from build123d import *

# Parameters (mm, degrees)
EXTRUDE_1_DEPTH     = 3
SKETCH_3_W          = 25
SKETCH_3_H          = 25
CUT_EXTRUDE_1_DEPTH = 391.157969373
SKETCH_5_R          = 1.5
CUT_EXTRUDE_3_DEPTH = 391.157969373
FILLET_2_R          = 10
SKETCH_6_R          = 1.5
CUT_EXTRUDE_6_DEPTH = 10
SKETCH_7_R          = 1.5
CUT_EXTRUDE_7_DEPTH = 391.157969373


with BuildPart() as part:
    # 草图1 → 凸台-拉伸1 (new body)
    with BuildSketch(Plane.XY):
        Polygon((0, -137.801455237), (0, 0), (-365, 0), (-365, -40), align=None)
    extrude(amount=EXTRUDE_1_DEPTH)

    # 草图3 → 切除-拉伸1 (cut, through all)
    with BuildSketch(Plane.XY.offset(3)):
        with Locations((-12.5, -12.5)):
            Rectangle(SKETCH_3_W, SKETCH_3_H)
    extrude(amount=-CUT_EXTRUDE_1_DEPTH, mode=Mode.SUBTRACT)

    # 草图5 → 切除-拉伸3 (cut, through all)
    with BuildSketch(Plane.XY.offset(3)):
        with Locations((-305, -7)):
            Circle(SKETCH_5_R)
        with Locations((-185, -7)):
            Circle(SKETCH_5_R)
        with Locations((-65, -7)):
            Circle(SKETCH_5_R)
    extrude(amount=-CUT_EXTRUDE_3_DEPTH, mode=Mode.SUBTRACT)

    # 圆角2
    fillet_2_edges = [part.edges().sort_by_distance(p)[0] for p in [
        (0, -25, 1.5),
        (-25, -25, 1.5),
        (-25, 0, 1.5),
    ]]
    fillet(fillet_2_edges, radius=FILLET_2_R)

    # 草图6 → 切除-拉伸6 (cut)
    with BuildSketch(Plane.XY.offset(3)):
        with Locations((-38.637033052, -119.16648399)):
            Circle(SKETCH_6_R)
        with Locations((-67.61480784, -111.401912637)):
            Circle(SKETCH_6_R)
        with Locations((-251.140714835, -62.226294067)):
            Circle(SKETCH_6_R)
        with Locations((-280.118489624, -54.461722714)):
            Circle(SKETCH_6_R)
    extrude(amount=-CUT_EXTRUDE_6_DEPTH, mode=Mode.SUBTRACT)

    # 草图7 → 切除-拉伸7 (cut, through all)
    with BuildSketch(Plane.XY.offset(3)):
        with Locations((-26.327035604, -95.030119084)):
            Circle(SKETCH_7_R)
        with Locations((-16.086178306, -77.850921146)):
            Circle(SKETCH_7_R)
    extrude(amount=-CUT_EXTRUDE_7_DEPTH, mode=Mode.SUBTRACT)


solid = part.part
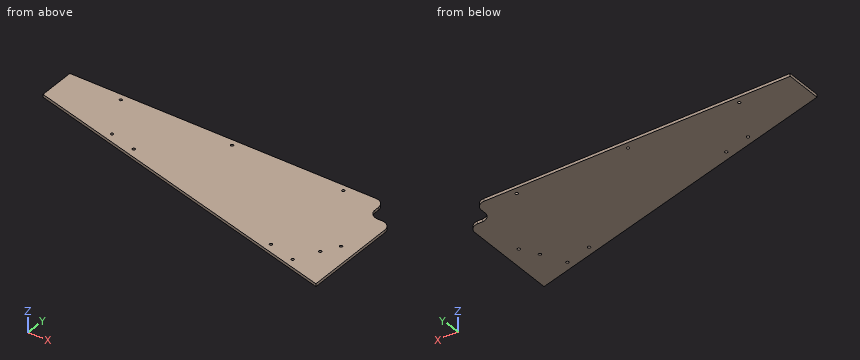
Build history of the part. All positions in model axes, mm. Round coordinates to 2 decimals unless told otherwise and drop trailing zeros. Order: outer loops, then holes, each group sorted by start corner. A loop starts at its lowest first (then second) coordinate and runs counter-clockwise, first axis right, second up. Notation, with made-up numbers: M 53,88.25 L 66,88.25 A22 cw 66,119.25 Z; hole C 54,-13 d9. An arc over 180 degrees is marked long. Use CSV: the item, a comma, the result in double quotes. Start each with the question number.
(1) Cut at C-C on x = -31.5. List the corners of the cut face in (y, z).
(2) Cut at B-B on y = -83.5. List the corners of the cut face in (x, z).
(3) Cut at A-A on z = 1.1. State how many separate pieces and enclosed holes the cut face has, then the cut area to 3 significant figures.
(4) Drill centre lines: probe 1 along X at (y, z) = (-17, 1.95); probe 2 along X at (y, z) = (-9, 1.15); probe 3 along Y at (x, z) = (-194.5, 1.1). Where is each one in solid material? Low to high.
(5) Flat gauge pin, fed straight in: P1, Ø1.5, axis at y = -28.5, z = 1.5, coming from the +X side. Where does the tip first touch, or does it go through?
Findings:
1,outline,"M -129.36,0 L -0.63,0 L -0.63,3 L -129.36,3 Z"
2,outline,"M -202.66,0 L 0,0 L 0,3 L -202.66,3 Z"
3,separate pieces,"1"
3,enclosed holes,"9"
3,area,"31,700 mm^2"
4,probe 1,"x = -365 to -24.8"
4,probe 2,"x = -365 to -25.05"
4,probe 3,"y = -85.69 to 0"
5,P1,"stops at x = -1.82"
